Input: part model. Units: mm. Frame: model coordinates. Round coordinates to 2 decimals unless told otherwise and drop trailing zeros. Order: outer loops, then holes, each group sorted by start corner. A loop starts at its lowest first (then second) coordinate and runs counter-clockwise, first axis right, second up. Notation, with made-up numbers: (-3, 39.5) -> (43, 39.5) arc R25 ccw to (43, 65.5) -> close; hole circle Ø11 at (69, 80.25). An arc over 180 degrees is marked (long way). Use a Markdown table: item, result.
from build123d import *

# Parameters (mm, degrees)
F2_SIZE = 0.2


# Not quite as in the source:
# - a feature names something its author has since deleted; it is built from what else it names


with BuildPart() as f1:
    # F0 (on Front) → F1 (revolve)
    with BuildSketch(Plane.XZ):
        with BuildLine():
            Line((0, 12.5), (0, 0))
            Line((0, 0), (0, -12.5))
            Line((0, -12.5), (1.25, -12.5))
            Line((1.25, -12.5), (1.25, -5.4047375097))
            ThreePointArc((1.25, -5.4047375097), (0.6905249807, -4), (0.5, -2.5))
            Line((0.5, -2.5), (0.5, 0))
            Line((0.5, 0), (0.5, 2.5))
            ThreePointArc((0.5, 2.5), (0.6905249807, 4), (1.25, 5.4047375097))
            Line((1.25, 5.4047375097), (1.25, 12.5))
            Line((1.25, 12.5), (0, 12.5))
        make_face()
    revolve(axis=Axis((0, 0, 6.25), (0, 0, 1)))

    # F2
    f2_edges = [f1.edges().sort_by_distance(p)[0] for p in [
        (-1.25, 0, -12.5),
        (-1.25, 0, 12.5),
    ]]
    chamfer(f2_edges, length=F2_SIZE)


solid = f1.part
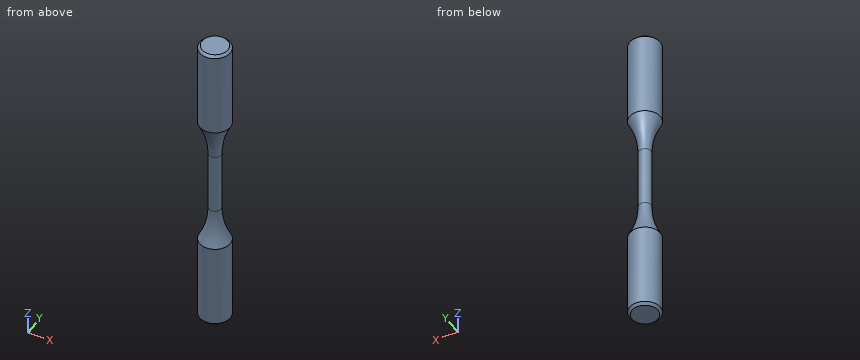
1) Cut plane C-C on z = 6.75. Return loops of the section in (x, y), and give its area (3 significant figures).
Results found:
| item | result |
|---|---|
| outline | circle Ø2.5 at (0, 0) |
| area | 4.91 mm² |
2) Line query: L1, parallel to X at y = -0.1, z = 9.5; L2, parallel to Z at x = 0.9, y = -0.3; L3, parallel to Z at x = 0.95, y = 0.35. Output: solid intervals per line, ascending. Write a range as [from, to].
Results found:
| item | result |
|---|---|
| L1 | x = [-1.25, 1.25] |
| L2 | z = [-12.5, -4.78], [4.78, 12.5] |
| L3 | z = [-12.5, -4.93], [4.93, 12.5] |
3) Cut plane D-D on z = -5. Return loops of the section in (x, y).
Results found:
| item | result |
|---|---|
| outline | circle Ø2.09 at (0, 0) |
4) Cut plane A-A on x = 0. Return loops of the section in (y, z), and give its area (3 significant figures).
Results found:
| item | result |
|---|---|
| outline | (-1.25, -12.3) -> (-1.05, -12.5) -> (1.05, -12.5) -> (1.25, -12.3) -> (1.25, -5.4) arc R6 cw to (0.5, -2.5) -> (0.5, 2.5) arc R6 cw to (1.25, 5.4) -> (1.25, 12.3) -> (1.05, 12.5) -> (-1.05, 12.5) -> (-1.25, 12.3) -> (-1.25, 5.4) arc R6 cw to (-0.5, 2.5) -> (-0.5, -2.5) arc R6 cw to (-1.25, -5.4) -> close |
| area | 49.0 mm² |
